The model under review builds one solid part; all positions refer to its coordinate system, in mm. A direction names the side the tool comes from. Coordinates: 2 decimals unless noted, no trailing zeros. Write each loop counter-clockwise with the first axis right and the second up, starting at its lowest first coordinate (ties: lowest second). Pieces come first, ordered by that corner, then holes. Notation, with made-up numbers: (-10.75, 42.25) -> (1.25, 42.25) arc R23 cw to (1.25, 55.25) -> close; hole circle Ø3 at (79.25, 8). An arc over 180 degrees is marked (long way). Put each result on its own line as item: value. Start each with the question number.
from build123d import *

# Parameters (mm, degrees)
SKETCH1_W                = 52
SKETCH1_H                = 24
SKETCH1_R                = 8.25
BOSS_EXTRUDE1_DEPTH      = 12
SKETCH2_R                = 1
CUT_EXTRUDE1_DEPTH       = 32.048349393
SKETCH3_R                = 1.75
CUT_EXTRUDE2_DEPTH       = 1
CUT_EXTRUDE3_DEPTH       = 5
FILLET3_R                = 0.5
CHAMFER1_SIZE            = 2.5
SKETCH5_W                = 19
SKETCH5_H                = 12
BOSS_EXTRUDE2_DEPTH      = 8
SKETCH6_W                = 7
SKETCH6_H                = 19
BOSS_EXTRUDE3_DEPTH      = 24
CHAMFER2_SIZE            = 3
CHAMFER2_OF_MIRROR1_SIZE = 3
SKETCH7_W                = 14
SKETCH7_H                = 8
CUT_EXTRUDE4_DEPTH       = 5
FILLET4_R                = 0.5
BOSS_EXTRUDE4_DEPTH      = 12
SKETCH9_W                = 26.398994769
SKETCH9_H                = 16
CUT_EXTRUDE5_DEPTH       = 13


with BuildPart() as part:
    # Sketch1 → Boss-Extrude1 (new body)
    with BuildSketch(Plane(origin=(0, 0, 0), x_dir=(1, 0, 0), z_dir=(0, 1, 0))):
        Rectangle(SKETCH1_W, SKETCH1_H)
        with Locations(Location((12.75, 0, 0), (0, 0, 270))):
            Circle(SKETCH1_R, mode=Mode.SUBTRACT)
        with Locations(Location((-12.75, 0, 0), (0, 0, 270))):
            Circle(SKETCH1_R, mode=Mode.SUBTRACT)
    extrude(amount=BOSS_EXTRUDE1_DEPTH)

    # Sketch2 → Cut-Extrude1 (cut, through all)
    with BuildSketch(Plane(origin=(0, 12, 0), x_dir=(1, 0, 0), z_dir=(0, 1, 0))):
        with Locations(Location((-21.35, 8.85, 0), (0, 0, 270))):
            Circle(SKETCH2_R)
        with Locations(Location((21.35, 8.85, 0), (0, 0, 270))):
            Circle(SKETCH2_R)
        with Locations(Location((21.35, -8.85, 0), (0, 0, 270))):
            Circle(SKETCH2_R)
        with Locations(Location((-21.35, -8.85, 0), (0, 0, 270))):
            Circle(SKETCH2_R)
    extrude(amount=-CUT_EXTRUDE1_DEPTH, mode=Mode.SUBTRACT)

    # Sketch3 → Cut-Extrude2 (cut)
    with BuildSketch(Plane(origin=(0, 12, 0), x_dir=(1, 0, 0), z_dir=(0, 1, 0))):
        with Locations(Location((-21.35, 8.85, 0), (0, 0, 270))):
            Circle(SKETCH3_R)
        with Locations(Location((21.35, 8.85, 0), (0, 0, 270))):
            Circle(SKETCH3_R)
        with Locations(Location((21.35, -8.85, 0), (0, 0, 270))):
            Circle(SKETCH3_R)
        with Locations(Location((-21.35, -8.85, 0), (0, 0, 270))):
            Circle(SKETCH3_R)
    extrude(amount=-CUT_EXTRUDE2_DEPTH, mode=Mode.SUBTRACT)

    # Sketch4 → Cut-Extrude3 (cut)
    with BuildSketch(Plane.XZ):
        Polygon((-6, -5), (-6, -12), (6, -12), (6, -5), (0, -5), align=None)
    extrude(amount=-CUT_EXTRUDE3_DEPTH, mode=Mode.SUBTRACT)

    # Fillet3
    fillet3_edges = [part.edges().sort_by_distance(p)[0] for p in [
        (-6, 2.5, -5),
        (6, 5, -8.5),
        (6, 2.5, -5),
        (-6, 5, -8.5),
        (0, 5, -5),
    ]]
    fillet(fillet3_edges, radius=FILLET3_R)

    # Chamfer1
    chamfer1_edges = [part.edges().sort_by_distance(p)[0] for p in [
        (26, 6, 12),
        (-26, 6, 12),
        (-26, 6, -12),
        (26, 6, -12),
    ]]
    chamfer(chamfer1_edges, length=CHAMFER1_SIZE)

    # Sketch5 → Boss-Extrude2 (add)
    with BuildSketch(Plane.ZY.offset(26)):
        with Locations((0, 6)):
            Rectangle(SKETCH5_W, SKETCH5_H)
    boss_extrude2 = extrude(amount=BOSS_EXTRUDE2_DEPTH)

    # Sketch6 → Boss-Extrude3 (add)
    with BuildSketch(Plane.XZ):
        with Locations((-30.5, 0)):
            Rectangle(SKETCH6_W, SKETCH6_H)
    boss_extrude3 = extrude(amount=BOSS_EXTRUDE3_DEPTH)

    # Chamfer2
    chamfer2_edges = [part.edges().sort_by_distance(p)[0] for p in [
        (-34, -6, 9.5),
        (-34, 12, 0),
        (-34, -6, -9.5),
    ]]
    chamfer(chamfer2_edges, length=CHAMFER2_SIZE)

    # Mirror1: Boss-Extrude2, Boss-Extrude3 across plane
    add(boss_extrude2.mirror(Plane(origin=(0, 0, 0), x_dir=(0, 0, 1), z_dir=(1, 0, 0))))
    add(boss_extrude3.mirror(Plane(origin=(0, 0, 0), x_dir=(0, 0, 1), z_dir=(1, 0, 0))))

    # Chamfer2 of Mirror1
    chamfer2_of_mirror1_edges = [part.edges().sort_by_distance(p)[0] for p in [
        (34, -6, 9.5),
        (34, 12, 0),
        (34, -6, -9.5),
    ]]
    chamfer(chamfer2_of_mirror1_edges, length=CHAMFER2_OF_MIRROR1_SIZE)

    # Sketch7 → Cut-Extrude4 (cut)
    with BuildSketch(Plane.XZ):
        with Locations((0, 12)):
            Rectangle(SKETCH7_W, SKETCH7_H)
    extrude(amount=-CUT_EXTRUDE4_DEPTH, mode=Mode.SUBTRACT)

    # Fillet4
    fillet4_edges = [part.edges().sort_by_distance(p)[0] for p in [
        (-7, 2.5, 8),
        (7, 5, 10),
        (0, 5, 8),
        (-7, 5, 10),
        (7, 2.5, 8),
    ]]
    fillet(fillet4_edges, radius=FILLET4_R)

    # Sketch8 → Boss-Extrude4 (add)
    with BuildSketch(Plane.XZ):
        Polygon((-7, 12), (7, 12), (23.5, 12), (26, 9.5), (27, 9.5), (27, -9.5), (26, -9.5), (23.5, -12), (6, -12), (-6, -12), (-23.5, -12), (-26, -9.5), (-27, -9.5), (-27, 9.5), (-26, 9.5), (-23.5, 12), align=None)
    extrude(amount=-BOSS_EXTRUDE4_DEPTH)

    # Sketch9 → Cut-Extrude5 (cut)
    with BuildSketch(Plane.XZ):
        with Locations((0.089665153, 4.133644411)):
            Rectangle(SKETCH9_W, SKETCH9_H)
    extrude(amount=-CUT_EXTRUDE5_DEPTH, mode=Mode.SUBTRACT)


solid = part.part
1. Wall thickness on line 1 (X direction, y = -4.5, z = 2.75); line 2 (X direction, y = 9, z = 1.75); line 3 (Y direction, x = 19, z = -4.75): over which ranges is each line inside the solid? List them lowest first. Write a range as from..to.
2. The part is to be moulded in two halves that separate along X. For faces 1 (the flat face through (32.5, -6.3, -8)), 2 (the flat face through (-27, -12, 0)), 3 (the flat face through (29, -6, 9.5)), say which applies: released by +X, released by -X, zero draft, split by the parting line, or undercut.
3. Consider section C-C on z = -8.75. State the section outline as (x, y) points.
4. Insertion check: P1, Ø1.5, axis at x = 29.5, y = -3.5, coming from the +Z side; P2, Ø8, axis at x = -15, y = -5, coming from the +Z side; P3, Ø1.5, axis at x = 27.5, y = -6.5, coming from the -Z side; P4, Ø5.5, axis at x = -28, y = 2.5, coming from the +Z side. Each pin has a flat end and moves straight along its axis. Give the tip position at first contact, or say it passes through.
5. Tool access review of faces 4 (the flat face through (-29, -6, 9.5)), 5 (the flat face through (-32, 11, 0)), 6 (the flat face through (27, -12, 0)), 7 (the flat face through (-34, -7, 0)), 8 (the flat face through (-13.11, 6, 4)): name each direction out of +Z, -Z, +X, -X, +Y, -Y from which nothing blocks a thin tool from reaching the whole face with its end or side.
6. Consider section A-A on y = -7. State the section outline as (x, z) points, then the cut area to 3 significant figures.
7. Consider section D-D on x = 24.5. State the section outline as (y, z) points.
8. Consider section B-B on z = 1. State the section outline as (x, y) points, then the cut area to 3 significant figures.
Output values:
1. line 1: x = -34..-27, 27..34
1. line 2: x = -34..-13.11, 13.29..34
1. line 3: y = 0..12
2. face 1: released by +X
2. face 2: undercut
2. face 3: zero draft
3. outline: (-31.75, -24) -> (-27, -24) -> (-27, 0) -> (27, 0) -> (27, -24) -> (31.75, -24) -> (31.75, 11.25) -> (31, 12) -> (-31, 12) -> (-31.75, 11.25) -> close
4. P1: stops at z = 9.5
4. P2: passes through
4. P3: stops at z = -9.5
4. P4: stops at z = 10.25
5. face 4: +Z, -X, +Y, -Y
5. face 5: +Z, -Z, -X, +Y
5. face 6: +Z, -Z, -Y
5. face 7: +Z, -Z, -X, +Y, -Y
5. face 8: +Z, +Y, -Y
6. outline: (-34, -6.5) -> (-31, -9.5) -> (-27, -9.5) -> (-27, 9.5) -> (-31, 9.5) -> (-34, 6.5) -> close; (27, -9.5) -> (31, -9.5) -> (34, -6.5) -> (34, 6.5) -> (31, 9.5) -> (27, 9.5) -> close
6. area: 248 mm^2
7. outline: (0, -11) -> (12, -11) -> (12, 11) -> (0, 11) -> close
8. outline: (-34, -24) -> (-27, -24) -> (-27, 0) -> (-13.11, 0) -> (-13.11, 12) -> (-31, 12) -> (-34, 9) -> close; (13.29, 0) -> (27, 0) -> (27, -24) -> (34, -24) -> (34, 9) -> (31, 12) -> (13.29, 12) -> close
8. area: 826 mm^2
